Input: part model. Units: mm. Frame: model coordinates. Face numbers are marked on the shaded views. A direction names the side the tool comes from. Coordinates: 2 decimals unless noted, no trailing zeros. Write each loop counter-clockwise with the first axis right and the second up, starting at its lowest first coordinate (ties: lowest second). Pieces come first, ordered by that corner, then holes. Notation, with made-up numbers: (17.25, 76.25) - (44.25, 76.25) arc R27 ccw to (44.25, 105.25) - close; hole circle Ø3 at (47.25, 50.25). An arc over 180 degrees is marked (long way). Put each result on its own line as item: value. Start each with the question number.
1. Cut plane B-B, the plane y = 22.5. Return loops of the section in (x, z), and give its area (3 significant figures).
2. Line query: line 1 (Y direction, x = 27, z = 2.75); line 2 (Y direction, x = -9.5, z = -0.5); line 3 (X direction, y = 0, z = 4). Output: solid intervals per line, ascending.
3. Pin query (flat end, axial travel): pin 1 (12 mm diameter, centred on x = 27.5, y = 18, fed in from +Z). Return the tip coordinate at first contact, or that it passes through.
4. Cut plane C-C, the plane x = 9.5. Return loops of the section in (y, z).
5. Cut plane D-D, the plane y = -9. Return loops of the section in (x, z), and give its area (3 significant figures).
6. Pull-direction query (X, two-part tool) for the marked faces 3, 4 and 5; classes: released by +X, released by -X, zero draft, split by the parting line, or undercut.
7. Cut plane A-A, the plane z = -1.75. Return loops of the section in (x, y).
8. Access query for the marked faces 1 and 2. Directions: +Z, -Z, +X, -X, +Y, -Y. A direction counts if a zero-diameter tool reaches every point of the face in a straight line with its end or side. Return the directions, or none.
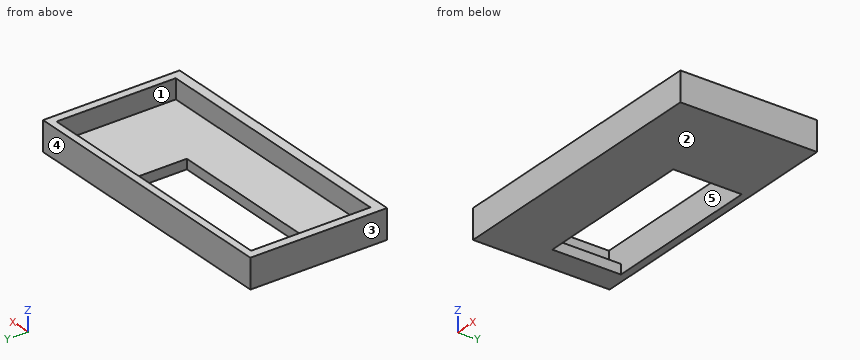
from build123d import *

# Parameters (mm, degrees)
SKETCH2_W           = 85.76635514
SKETCH2_H           = 41.829906542
SKETCH2_W_2         = 80.5
SKETCH2_H_2         = 36.5
BOSS_EXTRUDE1_DEPTH = 6
SKETCH4_W           = 85.76635514
SKETCH4_H           = 41.829906542
BOSS_EXTRUDE2_DEPTH = 3
SKETCH6_W           = 50
SKETCH6_H           = 21
CUT_EXTRUDE1_DEPTH  = 10


with BuildPart() as part:
    # Sketch2 → Boss-Extrude1 (new body)
    with BuildSketch(Plane.XY):
        with Locations((5.943457944, 7.071962617)):
            Rectangle(SKETCH2_W, SKETCH2_H)
        with Locations((6.018691589, 7.479906542)):
            Rectangle(SKETCH2_W_2, SKETCH2_H_2, mode=Mode.SUBTRACT)
    extrude(amount=BOSS_EXTRUDE1_DEPTH)

    # Sketch4 → Boss-Extrude2 (add)
    with BuildSketch(Plane(origin=(0, 0, 0), x_dir=(-1, 0, 0), z_dir=(0, 0, -1))):
        with Locations((-5.943457944, 7.071962617)):
            Rectangle(SKETCH4_W, SKETCH4_H)
    extrude(amount=BOSS_EXTRUDE2_DEPTH)

    # Sketch6 → Cut-Extrude1 (cut)
    with BuildSketch(Plane.XY):
        with Locations((-4.231308411, 15.229906542)):
            Rectangle(SKETCH6_W, SKETCH6_H)
    extrude(amount=-CUT_EXTRUDE1_DEPTH, mode=Mode.SUBTRACT)


solid = part.part
Report:
1. outline: (-36.94, -3) - (-29.23, -3) - (-29.23, 0) - (-34.23, 0) - (-34.23, 6) - (-36.94, 6) - close; (20.77, -3) - (48.83, -3) - (48.83, 6) - (46.27, 6) - (46.27, 0) - (20.77, 0) - close
1. area: 139 mm^2
2. line 1: y = -13.84 to -10.77, 25.73 to 27.99
2. line 2: y = -13.84 to 4.73, 25.73 to 27.99
2. line 3: x = -36.94 to -34.23, 46.27 to 48.83
3. pin 1: stops at z = 0
4. outline: (-13.84, -3) - (4.73, -3) - (4.73, 0) - (-10.77, 0) - (-10.77, 6) - (-13.84, 6) - close; (25.73, -3) - (27.99, -3) - (27.99, 6) - (25.73, 6) - close
5. outline: (-36.94, -3) - (48.83, -3) - (48.83, 6) - (46.27, 6) - (46.27, 0) - (-34.23, 0) - (-34.23, 6) - (-36.94, 6) - close
5. area: 289 mm^2
6. face 3: released by -X
6. face 4: zero draft
6. face 5: undercut
7. outline: (-36.94, -13.84) - (48.83, -13.84) - (48.83, 27.99) - (-36.94, 27.99) - close; hole (-29.23, 4.73) - (20.77, 4.73) - (20.77, 25.73) - (-29.23, 25.73) - close
8. face 1: +Z
8. face 2: -Z, +X, -X, +Y, -Y
